Geometry check sheet. Reference: the model listing, model coordinates, mm. Give positions to 0.01 mm unless a question says otherwise; leave off trailing zeros. Loops run counter-clockwise (first coordinate to the right, second up) from the corner with the lowest first, then second, coordinate; pieces in that order, holes last. Notation, with made-up numbers: (-33.5, 61.25) - (25.5, 61.25) arc R31 ccw to (25.5, 88.25) - close; hole circle Ø7 at (-22, 58). An arc over 180 degrees is marked (long way). Use a Markdown table: item, result. Add a question column.
1. Material ranges on L1, parallel to X at y = -67, z = -1.75; L2, parallel to Y at x = -56, z = -3.75; L3, parallel to Y at x = 70, z = 2.5, recorded low to high.
2. Cross-section at C-C on z = -2.5. Count the separate pieces of the cut face and the enclosed holes in it, and give its area (3 significant figures).
3. Cross-section at A-A on x = -55. Enter the section's corners in (y, z), and give its area (3 significant figures).
4. Cross-section at D-D on x = 85. Enter the section's corners in (y, z), and give its area (3 significant figures).
5. Depth check by flat-ended pin: P1, Ø2, axis at x = 102.5, z = 1, coming from the -Y side; P2, Ø2, axis at y = -76.5, z = 2.5, coming from the +X side; P3, Ø6, axis at x = -138, z = -1.5, coming from the +Y side. Enter the tip coordinate at first touch or a pass-through.
6. Cross-section at B-B on y = -110. Enter the section's corners in (x, z), and give its area (3 significant figures).
from build123d import *

# Parameters (mm, degrees)
BOSS_EXTRUDE1_DEPTH        = 6
F_7_0_7_DIAMETER_HOLE1_D   = 7
LPATTERN1_COUNT            = 4
LPATTERN1_PITCH            = 22
FILLET1_R                  = 5
MIRROR1_COPY_1_D           = 7
MIRROR1_COPY_2_D           = 7
MIRROR1_COPY_3_D           = 7
FILLET1_OF_MIRROR1_R       = 5
MIRROR5_COPY_1_D           = 7
MIRROR5_COPY_2_D           = 7
MIRROR5_COPY_3_D           = 7
FILLET1_OF_MIRROR5_R       = 5
MIRROR6_START              = -6
MIRROR6_OUTLINE_R          = 3.5
MIRROR6_DEPTH              = 12
F_6_8_6_8_DIAMETER_HOLE1_D = 6.8


# Read off the part's stored shape, not the designer's step: Mirror6
with BuildPart() as part:
    # Sketch1 → Boss-Extrude1 (new, symmetric)
    with BuildSketch(Plane.XY):
        with BuildLine():
            Line((0, 0), (0, 125))
            Line((0, 125), (34, 125))
            ThreePointArc((34, 125), (61.824855787, 57.824855787), (129, 30))
            Line((129, 30), (150, 30))
            Line((150, 30), (150, 0))
            Line((150, 0), (114.303256495, 0))
            Line((114.303256495, 0), (0, 0))
        make_face()
    boss_extrude1 = extrude(amount=BOSS_EXTRUDE1_DEPTH, both=True)

    # Ø7.0 (7) Diameter Hole1 (through all)
    with Locations(Plane.XY.offset(6)):
        with Locations((26, 110)):
            f_7_0_7_diameter_hole1 = Hole(F_7_0_7_DIAMETER_HOLE1_D / 2)

    # LPattern1: Ø7.0 (7) Diameter Hole1 ×4
    with Locations(*[(0, -i * LPATTERN1_PITCH, 0) for i in range(1, LPATTERN1_COUNT)]):
        add(f_7_0_7_diameter_hole1, mode=Mode.SUBTRACT)

    # Fillet1
    fillet1_edges = [part.edges().sort_by_distance(p)[0] for p in [
        (34, 125, 0),
        (150, 30, 0),
    ]]
    fillet(fillet1_edges, radius=FILLET1_R)

    # Mirror1: Boss-Extrude1, Ø7.0 (7) Diameter Hole1 across plane
    add(boss_extrude1.mirror(Plane(origin=(0, 0, 6), x_dir=(0, 0, 1), z_dir=(1, 0, 0))))
    add(f_7_0_7_diameter_hole1.mirror(Plane(origin=(0, 0, 6), x_dir=(0, 0, 1), z_dir=(1, 0, 0))), mode=Mode.SUBTRACT)

    # Mirror1 copy 1 (through all)
    with Locations(Plane(origin=(0, -22, 6), x_dir=(-1, 0, 0), z_dir=(0, 0, 1))):
        with Locations((26, -110)):
            Hole(MIRROR1_COPY_1_D / 2)

    # Mirror1 copy 2 (through all)
    with Locations(Plane(origin=(0, -44, 6), x_dir=(-1, 0, 0), z_dir=(0, 0, 1))):
        with Locations((26, -110)):
            Hole(MIRROR1_COPY_2_D / 2)

    # Mirror1 copy 3 (through all)
    with Locations(Plane(origin=(0, -66, 6), x_dir=(-1, 0, 0), z_dir=(0, 0, 1))):
        with Locations((26, -110)):
            Hole(MIRROR1_COPY_3_D / 2)

    # Fillet1 of Mirror1
    fillet1_of_mirror1_edges = [part.edges().sort_by_distance(p)[0] for p in [
        (-34, 125, 0),
        (-150, 30, 0),
    ]]
    fillet(fillet1_of_mirror1_edges, radius=FILLET1_OF_MIRROR1_R)

    # Mirror5: Boss-Extrude1, Ø7.0 (7) Diameter Hole1 across plane
    add(boss_extrude1.mirror(Plane.ZX))
    add(f_7_0_7_diameter_hole1.mirror(Plane.ZX), mode=Mode.SUBTRACT)

    # Mirror5 copy 1 (through all)
    with Locations(Plane(origin=(0, 22, 6), x_dir=(1, 0, 0), z_dir=(0, 0, 1))):
        with Locations((26, -110)):
            Hole(MIRROR5_COPY_1_D / 2)

    # Mirror5 copy 2 (through all)
    with Locations(Plane(origin=(0, 44, 6), x_dir=(1, 0, 0), z_dir=(0, 0, 1))):
        with Locations((26, -110)):
            Hole(MIRROR5_COPY_2_D / 2)

    # Mirror5 copy 3 (through all)
    with Locations(Plane(origin=(0, 66, 6), x_dir=(1, 0, 0), z_dir=(0, 0, 1))):
        with Locations((26, -110)):
            Hole(MIRROR5_COPY_3_D / 2)

    # Fillet1 of Mirror5
    fillet1_of_mirror5_edges = [part.edges().sort_by_distance(p)[0] for p in [
        (34, -125, 0),
        (150, -30, 0),
    ]]
    fillet(fillet1_of_mirror5_edges, radius=FILLET1_OF_MIRROR5_R)

    # Mirror6 outline → Mirror6 (add)
    with BuildSketch(Plane.XY.offset(MIRROR6_START)):
        with BuildLine():
            Line((0, 0), (-150, 0))
            Line((-150, 0), (-150, -25))
            ThreePointArc((-150, -25), (-148.535533906, -28.535533906), (-145, -30))
            Line((-145, -30), (-129, -30))
            ThreePointArc((-129, -30), (-63.525768428, -56.165960456), (-34.118824312, -120.25))
            ThreePointArc((-34.118824312, -120.25), (-32.571090411, -123.622844187), (-29.125078223, -125))
            Line((-29.125078223, -125), (0, -125))
            Line((0, -125), (0, 0))
        make_face()
        with Locations((-26, -110)):
            Circle(MIRROR6_OUTLINE_R, mode=Mode.SUBTRACT)
        with Locations((-26, -88)):
            Circle(MIRROR6_OUTLINE_R, mode=Mode.SUBTRACT)
        with Locations((-26, -66)):
            Circle(MIRROR6_OUTLINE_R, mode=Mode.SUBTRACT)
        with Locations((-26, -44)):
            Circle(MIRROR6_OUTLINE_R, mode=Mode.SUBTRACT)
    extrude(amount=MIRROR6_DEPTH)

    # Ø6.8 (6.8) Diameter Hole1 (through all)
    with Locations(Plane.XY.offset(6)):
        with Locations((130, 15), (100, 15), (70, 15), (115, -15), (85, -15), (55, -15)):
            f_6_8_6_8_diameter_hole1 = Hole(F_6_8_6_8_DIAMETER_HOLE1_D / 2)

    # Mirror7: Ø6.8 (6.8) Diameter Hole1 across plane
    add(f_6_8_6_8_diameter_hole1.mirror(Plane(origin=(0, 0, 0), x_dir=(0, 0, 1), z_dir=(1, 0, 0))), mode=Mode.SUBTRACT)


solid = part.part
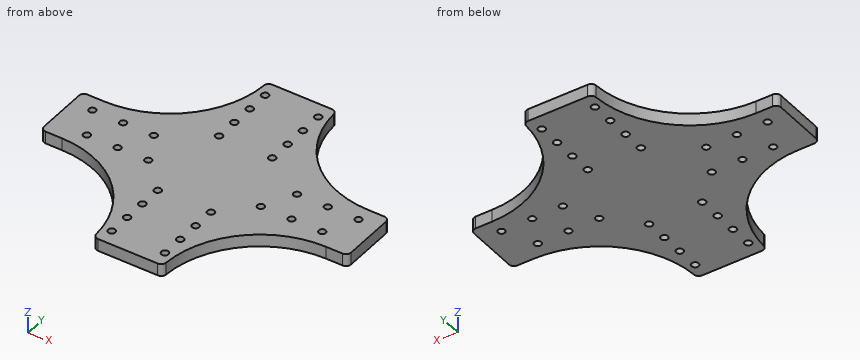
Values found:
| question | item | result |
|---|---|---|
| 1 | L1 | x = -53.76 to -29.35, -22.65 to 22.65, 29.35 to 53.76 |
| 1 | L2 | y = -64.21 to -18.25, -11.75 to 64.21 |
| 1 | L3 | y = -50.54 to 11.6, 18.4 to 50.54 |
| 2 | separate pieces | 1 |
| 2 | enclosed holes | 28 |
| 2 | area | 37,600 mm2 |
| 3 | outline | (-65.43, -6) - (-18.4, -6) - (-18.4, 6) - (-65.43, 6) - close; (-11.6, -6) - (65.43, -6) - (65.43, 6) - (-11.6, 6) - close |
| 3 | area | 1,490 mm2 |
| 4 | outline | (-40.8, -6) - (-18.4, -6) - (-18.4, 6) - (-40.8, 6) - close; (-11.6, -6) - (40.8, -6) - (40.8, 6) - (-11.6, 6) - close |
| 4 | area | 898 mm2 |
| 5 | P1 | stops at y = -34.07 |
| 5 | P2 | stops at x = 47.92 |
| 5 | P3 | stops at y = 30 |
| 6 | outline | (-35.19, -6) - (-29.5, -6) - (-29.5, 6) - (-35.19, 6) - close; (-22.5, -6) - (22.5, -6) - (22.5, 6) - (-22.5, 6) - close; (29.5, -6) - (35.19, -6) - (35.19, 6) - (29.5, 6) - close |
| 6 | area | 677 mm2 |
